Verification items for this drawing (mm, ordinates from the low corner). Round coordinates to 2 decimals unless told otherwise and drop trailing zeros. Loops run counter-clockwise (first coordinate to the right, second up) from the corner with the lowest first, then second, coordinate; pieces in that order, holes last. Notation, with made-up numbers: (76.5, 11) - (92.5, 11) arc R33 ccw to (92.5, 44) - close; hole circle Ø11 at (15.5, 0.25). An arc over 180 degrees is marked (long way). Put each result on its own line as item: value.
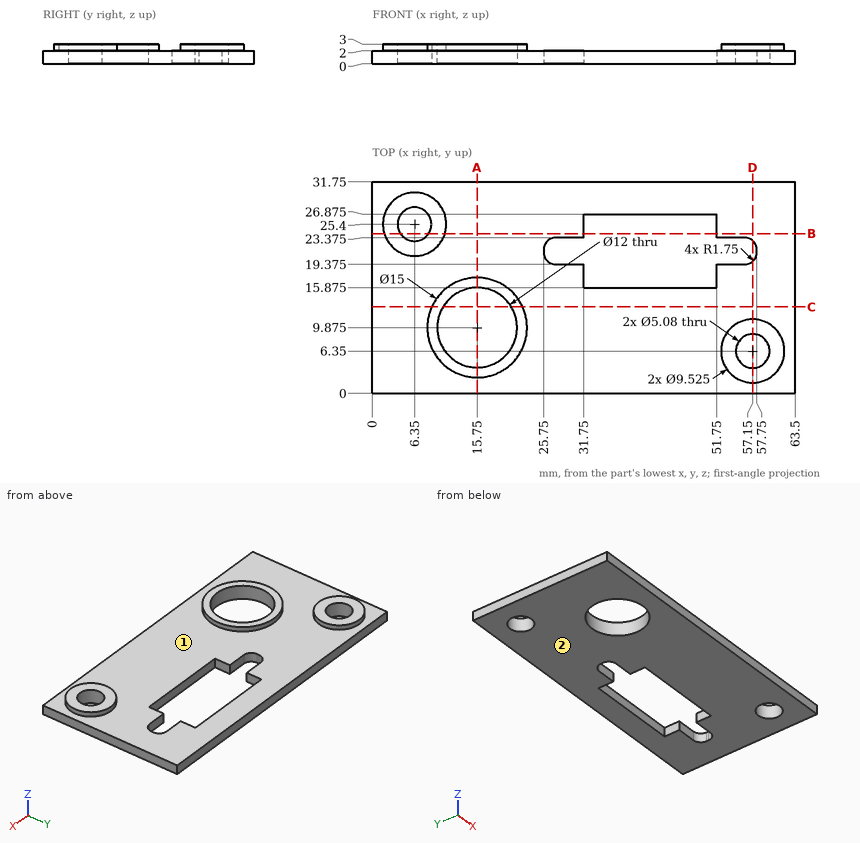
Item 1: Section check C-C on y = 13. Enter the section's corners in (x, z).
Filled sheet:
outline: (0, 0) - (10.63, 0) - (10.63, 3) - (8.93, 3) - (8.93, 2) - (0, 2) - close; (20.87, 0) - (63.5, 0) - (63.5, 2) - (22.57, 2) - (22.57, 3) - (20.87, 3) - close
Item 2: Section check D-D on x = 57.15. Enter the section's corners in (y, z).
Filled sheet:
outline: (0, 0) - (3.81, 0) - (3.81, 3) - (1.59, 3) - (1.59, 2) - (0, 2) - close; (8.89, 0) - (19.81, 0) - (19.81, 2) - (11.11, 2) - (11.11, 3) - (8.89, 3) - close; (22.94, 0) - (31.75, 0) - (31.75, 2) - (22.94, 2) - close
Item 3: Section check A-A on x = 15.75. Enter the section's corners in (y, z) (3 decimals).
Filled sheet:
outline: (0, 0) - (3.875, 0) - (3.875, 3) - (2.375, 3) - (2.375, 2) - (0, 2) - close; (15.875, 0) - (31.75, 0) - (31.75, 2) - (17.375, 2) - (17.375, 3) - (15.875, 3) - close
Item 4: Thickness scan on line 1 (Y direction, x = 36, z = 0.15) (3 decimals); line 2 (X direction, y = 21.5, z = 0.3); line 3 (Y direction, x = 6.35, z = 0.9). Record the ranges inside material, lowest first. Write a range as from..to.
Filled sheet:
line 1: 0..15.875, 26.875..31.75
line 2: 0..25.75, 57.75..63.5
line 3: 0..22.86, 27.94..31.75
Item 5: Go/stop test with flat-tipped pins: pin 1 (1.6 mm diameter, centred on y = 18.5, z = 1, fed in from -X); pin 2 (4.5 mm diameter, centred on x = 57.15, y = 6.35, fed in from -Z). Record where each tip stops, or that it passes through.
Filled sheet:
pin 1: x = 0
pin 2: through
Item 6: Release check for a two-part mould opening along Z. For the marked faces 1 and 2 record: +Z half, -Z half, draft (parallel to the pull), parting line (faces both ways), or undercut.
Filled sheet:
face 1: +Z half
face 2: -Z half
Item 7: Section check B-B on y = 24. Enter the section's corners in (x, z).
Filled sheet:
outline: (0, 0) - (4.23, 0) - (4.23, 3) - (1.8, 3) - (1.8, 2) - (0, 2) - close; (8.47, 0) - (31.75, 0) - (31.75, 2) - (10.9, 2) - (10.9, 3) - (8.47, 3) - close; (51.75, 0) - (63.5, 0) - (63.5, 2) - (51.75, 2) - close
